Geometry check sheet. Reference: the model listing, model coordinates, mm. Round coordinates to 2 decimals unless told otherwise and drop trailing zeros.
```python
from build123d import *

# Parameters (mm, degrees)
SKETCH1_W           = 12.7
SKETCH1_H           = 19.05
SKETCH1_W_2         = 3.175
SKETCH1_H_2         = 12.7
BOSS_EXTRUDE1_DEPTH = 457.2
BOSS_EXTRUDE2_REACH = 459.368
SKETCH2_R           = 3.175
SKETCH3_R           = 3.175
BOSS_EXTRUDE3_DEPTH = 6.35
BOSS_EXTRUDE4_START = 6.35
SKETCH4_R           = 3.175
BOSS_EXTRUDE4_DEPTH = 6.35


with BuildPart() as part:
    # Sketch1 → Boss-Extrude1 (new body)
    with BuildSketch(Plane(origin=(0, 0, 0), x_dir=(1, 0, 0), z_dir=(0, 1, 0))):
        Rectangle(SKETCH1_W, SKETCH1_H)
        Rectangle(SKETCH1_W_2, SKETCH1_H_2, mode=Mode.SUBTRACT)
    extrude(amount=BOSS_EXTRUDE1_DEPTH)

    # Sketch2 → Boss-Extrude2 (add, up to next)
    with BuildSketch(Plane(origin=(-1.5875, 0, 0), x_dir=(0, 0, -1), z_dir=(1, 0, 0)), mode=Mode.PRIVATE) as boss_extrude2_sk1:
        with Locations(Location((0, 450.85, 0), (0, 0, 180))):
            Circle(SKETCH2_R)
    boss_extrude2_tool1 = extrude(boss_extrude2_sk1.sketch, amount=BOSS_EXTRUDE2_REACH, mode=Mode.PRIVATE) - part.part
    add(boss_extrude2_tool1.solids().sort_by_distance((-1.5875, 450.85, 0))[0])

    # Sketch3 → Boss-Extrude3 (add)
    with BuildSketch(Plane(origin=(6.35, 0, 0), x_dir=(0, 0, -1), z_dir=(1, 0, 0))):
        with Locations(Location((0, 6.35, 0), (0, 0, 180))):
            Circle(SKETCH3_R)
    extrude(amount=BOSS_EXTRUDE3_DEPTH)

    # Sketch4 → Boss-Extrude4 (add)
    with BuildSketch(Plane.ZY.offset(6.35).offset(BOSS_EXTRUDE4_START)):
        with Locations((0, 6.35)):
            Circle(SKETCH4_R)
    extrude(amount=-BOSS_EXTRUDE4_DEPTH)


solid = part.part
```
1) Scan lines: line 1 along X through (y, z) = (317, -1.5); line 2 along Z through (x, y) = (0, 60) (3 decimals); line 3 along X through (y, z) = (436.5, 8). Record each from-to range of solid material in increasing order.
Report:
line 1: x = -6.35 to -1.59, 1.59 to 6.35
line 2: z = -9.525 to -6.35, 6.35 to 9.525
line 3: x = -6.35 to 6.35
2) Mould release check, pull along Z, two halves, no side actions. Record for faces 1 (the face through (0, 225, -9.525)), 2 (the face through (1.588, 225, 0)), 3 (the face through (6.35, 225, 0)): +Z half, -Z half, draft (parallel to the pull), parting line (faces both ways), or undercut.
Report:
face 1: -Z half
face 2: undercut
face 3: draft
3) Gauge pin test, flat ends, axial feed: pin 1 (4 mm diameter, centred on y = 329, z = -2.5, fed in from +X); pin 2 (2 mm diameter, centred on x = 7, z = -6, fed in from -Y); pin 3 (2 mm diameter, centred on y = 232.5, z = 5, fed in from -X). Record the tip position at first contact, or that the pin passes through.
Report:
pin 1: stops at x = 6.35
pin 2: stops at y = 0
pin 3: stops at x = -6.35
